from build123d import *

# Parameters (mm, degrees)
F0_W      = 25
F0_H      = 35
F1_DEPTH  = 4
F2_R      = 1.675
F3_DEPTH  = 25
F4_W      = 25
F4_H      = 11
F5_DEPTH  = 13
F7_DEPTH  = 6
F8_R      = 8
F9_DEPTH  = 5
F2_R_2    = 3
F10_DEPTH = 2
F11_R     = 5
F12_W     = 11
F12_H     = 17
F13_DEPTH = 2
F14_W     = 11
F14_H     = 17
F15_DEPTH = 2
F16_R     = 1.45
F17_DEPTH = 25
F18_R     = 4


with BuildPart() as f1:
    # F0 (on Top) → F1 (new body)
    with BuildSketch(Plane.XY):
        with Locations((12.5, 17.5)):
            Rectangle(F0_W, F0_H)
    extrude(amount=F1_DEPTH)

    # F2 (on face) → F3 (cut)
    with BuildSketch(Plane.XY.offset(4)):
        with BuildLine():
            ThreePointArc((3.325, 18.5605346784), (5, 16.8855346784), (6.675, 18.5605346784))
            ThreePointArc((6.675, 18.5605346784), (5, 20.2355346784), (3.325, 18.5605346784))
        make_face()
        with Locations((20, 18.5605346784)):
            Circle(F2_R)
        with Locations((20, 3.5605346784)):
            Circle(F2_R)
        with Locations((5, 3.5605346784)):
            Circle(F2_R)
    extrude(amount=-F3_DEPTH, mode=Mode.SUBTRACT)

    # F4 (on face) → F5 (join)
    with BuildSketch(Plane.XY.offset(4)):
        with Locations((12.5, 29.5)):
            Rectangle(F4_W, F4_H)
    extrude(amount=F5_DEPTH)

    # F6 (on face) → F7 (cut)
    with BuildSketch(Plane(origin=(0, 35, 0), x_dir=(-1, 0, 0), z_dir=(0, 1, 0))):
        with BuildLine():
            ThreePointArc((-18.5, 17), (-12.5, 11), (-6.5, 17))
            Line((-6.5, 17), (-18.5, 17))
        make_face()
    extrude(amount=-F7_DEPTH, mode=Mode.SUBTRACT)

    # F8 (on face) → F9 (cut)
    with BuildSketch(Plane.XZ.offset(-24)):
        with Locations((12.5, 17)):
            Circle(F8_R)
    extrude(amount=-F9_DEPTH, mode=Mode.SUBTRACT)

    # F2 (on face) → F10 (cut)
    with BuildSketch(Plane.XY.offset(4)):
        with BuildLine():
            ThreePointArc((8, 18.5605346784), (5, 21.5605346784), (2, 18.5605346784))
            ThreePointArc((2, 18.5605346784), (5, 15.5605346784), (8, 18.5605346784))
        make_face()
        with BuildLine():
            ThreePointArc((3.325, 18.5605346784), (5, 20.2355346784), (6.675, 18.5605346784))
            ThreePointArc((6.675, 18.5605346784), (5, 16.8855346784), (3.325, 18.5605346784))
        make_face(mode=Mode.SUBTRACT)
        with Locations((20, 18.5605346784)):
            Circle(F2_R_2)
        with Locations((20, 18.5605346784)):
            Circle(F2_R, mode=Mode.SUBTRACT)
        with Locations((20, 3.5605346784)):
            Circle(F2_R_2)
        with Locations((20, 3.5605346784)):
            Circle(F2_R, mode=Mode.SUBTRACT)
        with Locations((5, 3.5605346784)):
            Circle(F2_R_2)
        with Locations((5, 3.5605346784)):
            Circle(F2_R, mode=Mode.SUBTRACT)
    extrude(amount=-F10_DEPTH, mode=Mode.SUBTRACT)

    # F11
    f11_edges = [f1.edges().sort_by_distance(p)[0] for p in [
        (0, 0, 2),
        (25, 0, 2),
    ]]
    fillet(f11_edges, radius=F11_R)

    # F12 (on face) → F13 (join)
    with BuildSketch(Plane(origin=(0, 0, 0), x_dir=(0, -1, 0), z_dir=(-1, 0, 0))):
        with Locations((-29.5, 8.5)):
            Rectangle(F12_W, F12_H)
    extrude(amount=F13_DEPTH)

    # F14 (on face) → F15 (join)
    with BuildSketch(Plane.YZ.offset(25)):
        with Locations((29.5, 8.5)):
            Rectangle(F14_W, F14_H)
    extrude(amount=F15_DEPTH)

    # F16 (on face) → F17 (cut)
    with BuildSketch(Plane.XY.offset(17)):
        with Locations((0.45, 30.55)):
            Circle(F16_R)
        with Locations((24.55, 30.55)):
            Circle(F16_R)
    extrude(amount=-F17_DEPTH, mode=Mode.SUBTRACT)

    # F18
    f18_edges = [f1.edges().sort_by_distance(p)[0] for p in [
        (-2, 24, 8.5),
        (-2, 35, 8.5),
        (27, 35, 8.5),
        (27, 24, 8.5),
    ]]
    fillet(f18_edges, radius=F18_R)


solid = f1.part
Input: part model. Units: mm. Frame: model coordinates. A direction names the side the tool comes from. Coordinates: 2 decimals unless noted, no trailing zeros. Loops run counter-clockwise (first coordinate to the right, second up) from the corner with the lowest first, then second, coordinate; pieces in that order, holes last.
(1) Material intervals for probe 1 along Y at (x, z) = (20, 1.35); probe 2 along Y at (x, z) = (20, 3.3); probe 3 along X at (y, z) = (14, 2.25), sorted ascending.
(2) Section B-B on z = 6.5. Return the cut outline in (x, y).
(3) Section D-D on x = 12.5. Return the cut outline in (y, z).
(4) Set-up query: faces 1 (the face through (0, 15, 2)), 2 (the face through (4.35, 0.63, 3.01)), 3 (the face through (12, 35, 6)), 4 (the face through (12, 24, 8)). Return all of +Z, -Z, +X, -X, +Y, -Y with unobstructed straight access to the full face (end or side cutting, diameter ignored); none if empty.
(5) First-contact query: pin 1 Ø5 at (x, y) = (6.5, 20) entering from +Z; pin 2 Ø4 at (x, z) = (7.5, 10) entering from -Y; pin 3 Ø3 at (y, z) = (13.5, 2) entering from +X. Flat tips, straight axial feed; report the tip coordinate or a pass-through.
(6) Section C-C on x = 0.45. Return the cut outline in (y, z).
(7) Section A-A on y = 30.55. Return the cut outline in (x, z), then the cut area to 3 significant figures.
Data:
1. probe 1: y = 0 to 1.89, 5.24 to 16.89, 20.24 to 35
1. probe 2: y = 0 to 0.56, 6.56 to 15.56, 21.56 to 35
1. probe 3: x = 0 to 25
2. outline: (-2, 28) arc R4 ccw to (2, 24) - (23, 24) arc R4 ccw to (27, 28) - (27, 31) arc R4 ccw to (23, 35) - (2, 35) arc R4 ccw to (-2, 31) - close; hole circle Ø2.9 at (0.45, 30.55); hole circle Ø2.9 at (24.55, 30.55)
3. outline: (0, 0) - (35, 0) - (35, 11) - (29, 11) - (29, 9) - (24, 9) - (24, 4) - (0, 4) - close
4. face 1: +Z, -Z, -X, -Y
4. face 2: +Z
4. face 3: +Z, -Z, +X, -X, +Y
4. face 4: +Z, +X, -X, -Y
5. pin 1: stops at z = 4
5. pin 2: stops at y = 24
5. pin 3: stops at x = 25
6. outline: (2.93, 0) - (29.1, 0) - (29.1, 17) - (24.31, 17) - (24.31, 4) - (2.93, 4) - close; (32, 0) - (34.69, 0) - (34.69, 17) - (32, 17) - close
7. outline: (-2, 0) - (-1, 0) - (-1, 17) - (-2, 17) - close; (1.9, 0) - (23.1, 0) - (23.1, 17) - (18.5, 17) arc R6 cw to (6.5, 17) - (1.9, 17) - close; (26, 0) - (27, 0) - (27, 17) - (26, 17) - close
7. area: 338 mm2
